Autodesk Inventor part; units mm, degrees
ref_plane "YZ Plane" through (0, 0, 0) normal (1, 0, 0) x (0, 1, 0)
ref_plane "XZ Plane" through (0, 0, 0) normal (0, 1, 0) x (-1, 0, 0)
ref_plane "XY Plane" through (0, 0, 0) normal (0, 0, 1) x (1, 0, 0)
sketch "Sketch1" plane through (0, 0, 0) normal (0, 0, 1) x (1, 0, 0)
  line L0 (-73.5219, 27.2789) -> (440.7773, 27.2789)
  line L1 (440.7773, 27.2789) -> (440.7773, -861.7211)
  line L2 (440.7773, -861.7211) -> (-73.5219, -861.7211)
  line L3 (-73.5219, -861.7211) -> (-73.5219, 27.2789)
  point P0 (0, 0)
  dimension "d0" = 514.2992
  dimension "d1" = 889
extrude "Extrusion1" add sketch "Sketch1" along normal blind 6.35
sketch "Sketch3" plane through (0, 0, 6.35) normal (0, 0, 1) x (1, 0, 0)
  line L0 (-73.5219, 27.2789) -> (104.2781, 27.2789)
  line L1 (104.2781, 27.2789) -> (104.2781, -433.4771)
  line L2 (104.2781, -433.4771) -> (-73.5219, -433.4771)
  line L3 (-73.5219, -433.4771) -> (-73.5219, 27.2789)
  line L4 (440.7773, 27.2789) -> (262.9773, 27.2789)
  line L5 (262.9773, 27.2789) -> (262.9773, -433.4771)
  line L6 (262.9773, -433.4771) -> (440.7773, -433.4771)
  line L7 (440.7773, -433.4771) -> (440.7773, 27.2789)
  point P0 (0, 0)
  dimension "d4" = 177.8
  dimension "d5" = 460.756
  dimension "d6" = 177.8
  dimension "d7" = 460.756
extrude "Extrusion2" cut sketch "Sketch3" against normal blind 25.4
sketch "Sketch4" plane through (104.2781, 27.2789, 0) normal (0, 1, 0) x (1, 0, 0)
  line L0 (0, 0) -> (0, -6.35)
  line L1 (0, -6.35) -> (158.6992, -6.35)
  line L2 (158.6992, -6.35) -> (158.6992, 0)
  line L3 (0, 0) -> (158.6992, 0)
  point P0 (-104.2781, 0)
extrude "Extrusion3" add sketch "Sketch4" along normal blind 6.35
sketch "Sketch5" plane through (104.2781, 33.6289, 0) normal (0, 1, 0) x (1, 0, 0)
  line L0 (0, 0) -> (158.6992, 0)
  line L1 (0, -6.35) -> (0, 0)
  line L2 (158.6992, -6.35) -> (0, -6.35)
  line L3 (158.6992, 0) -> (158.6992, -6.35)
  point P0 (-104.2781, 0)
extrude "Extrusion4" cut sketch "Sketch5" against normal blind 6.35
sketch "Sketch6" plane through (104.2781, 27.2789, 0) normal (0, 1, 0) x (1, 0, 0)
  line L0 (0, -6.35) -> (0, 0)
  line L1 (158.6992, -6.35) -> (0, -6.35)
  line L2 (158.6992, 0) -> (158.6992, -6.35)
  line L3 (0, 0) -> (158.6992, 0)
  point P0 (-104.2781, 0)
extrude "Extrusion5" add sketch "Sketch6" along normal blind 6.35
sketch "Sketch7" plane through (0, 0, 0) normal (0, 0, -1) x (-1, 0, 0)
  line L0 (-440.7773, -861.7211) -> (73.5219, -861.7211)
  line L1 (-104.2781, 33.6289) -> (-262.9773, 33.6289)
  line L2 (-183.6277, -861.7211) -> (-183.6277, -362.9159)
  circle A0 centre (-183.6277, -362.9159) radius 2.3495
  point P0 (0, 0)
  dimension "d16" = 498.8052
  dimension "d17" = 4.699
extrude "Extrusion6" cut sketch "Sketch7" against normal blind 25.4
sketch "Sketch8" plane through (0, 0, 0) normal (0, 0, -1) x (-1, 0, 0)
  circle A0 centre (-183.6277, -362.9159) radius 2.3495
  line L0 (-104.2781, 33.6289) -> (-262.9773, 33.6289)
  line L1 (-183.6277, -362.9159) -> (-183.6277, -593.4209)
  circle A1 centre (-183.6277, -593.4209) radius 2.3495
  point P0 (0, 0)
  dimension "d20" = 230.505
  dimension "d21" = 4.699
extrude "Extrusion7" cut sketch "Sketch8" against normal blind 25.4 contours A1
sketch "Sketch9" plane through (0, 0, 0) normal (0, 0, -1) x (-1, 0, 0)
  circle A0 centre (-183.6277, -593.4209) radius 2.3495
  circle A1 centre (-183.6277, -362.9159) radius 2.3495
  line L0 (-104.2781, 33.6289) -> (-262.9773, 33.6289)
  line L1 (-183.6277, 33.6289) -> (-183.6277, -347.3711)
  circle A2 centre (-183.6277, -347.3711) radius 2.3495
  line L2 (-183.6277, -347.3711) -> (-183.6277, -362.9159)
  line L3 (-183.6277, -593.4209) -> (-183.6277, -577.8761)
  circle A3 centre (-183.6277, -577.8761) radius 2.3495
  point P0 (0, 0)
  dimension "d24" = 381
  dimension "d25" = 15.5448
extrude "Extrusion8" cut sketch "Sketch9" against normal blind 25.4 contours A3 | A2 L1 L2 | L2 L1 A2
sketch "Sketch10" plane through (0, 0, 0) normal (0, 0, -1) x (-1, 0, 0)
  circle A0 centre (-183.6277, -593.4209) radius 2.3495
  circle A1 centre (-183.6277, -362.9159) radius 2.3495
  point P0 (0, 0)
extrude "Extrusion9" add sketch "Sketch10" against normal blind 6.35
sketch "Sketch11" plane through (0, 0, 6.35) normal (0, 0, 1) x (1, 0, 0)
  line L0 (104.2781, -433.4771) -> (-73.5219, -433.4771)
  line L1 (-73.5219, -861.7211) -> (-73.5219, -433.4771)
  line L2 (440.7773, -861.7211) -> (-73.5219, -861.7211)
  line L3 (440.7773, -433.4771) -> (440.7773, -861.7211)
  line L4 (262.9773, 33.6289) -> (104.2781, 33.6289)
  line L5 (49.7648, -433.4771) -> (49.7648, -750.9771)
  line L6 (49.7648, -750.9771) -> (49.7648, -757.3271)
  line L7 (49.7648, -757.3271) -> (-73.5219, -757.3271)
  line L8 (49.7648, -757.3271) -> (440.7773, -757.3271)
  point P0 (0, 0)
  dimension "d30" = 317.5
  dimension "d31" = 6.35
extrude "Extrusion10" cut sketch "Sketch11" against normal blind 6.35 contours L7 L8 L3 L2 L1
sketch "Sketch12" plane through (0, 0, 0) normal (0, 0, -1) x (-1, 0, 0)
  line L0 (-440.7773, -433.4771) -> (-440.7773, -757.3271)
  circle A0 centre (-183.6277, -577.8761) radius 2.3495
  circle A1 centre (-183.6277, -347.3711) radius 2.3495
  line L1 (-183.6277, -347.3711) -> (-183.6277, -249.3271)
  line L2 (-183.6277, -577.8761) -> (-183.6277, -479.8321)
  circle A2 centre (-183.6277, -479.8321) radius 2.3495
  circle A3 centre (-183.6277, -249.3271) radius 2.3495
  point P0 (0, 0)
  dimension "d34" = 98.044
  dimension "d35" = 98.044
extrude "Extrusion11" cut sketch "Sketch12" against normal blind 6.35 contours A2 | A3
sketch "Sketch13" plane through (0, 0, 0) normal (0, 0, -1) x (-1, 0, 0)
  circle A0 centre (-183.6277, -577.8761) radius 2.3495
  circle A1 centre (-183.6277, -347.3711) radius 2.3495
  point P0 (0, 0)
extrude "Extrusion12" add sketch "Sketch13" against normal blind 6.35
sketch "Sketch14" plane through (0, 0, 6.35) normal (0, 0, 1) x (1, 0, 0)
  line L0 (262.9773, -433.4771) -> (262.9773, 33.6289)
  line L1 (104.2781, 33.6289) -> (262.9773, 33.6289)
  line L2 (262.9773, 33.6289) -> (262.9773, 14.5789)
  line L3 (262.9773, 14.5789) -> (104.2781, 14.5789)
  line L4 (104.2781, 14.5789) -> (104.2781, 33.6289)
  point P0 (0, 0)
  dimension "d40" = 19.05
extrude "Extrusion13" cut sketch "Sketch14" against normal blind 25.4
properties part number "front"
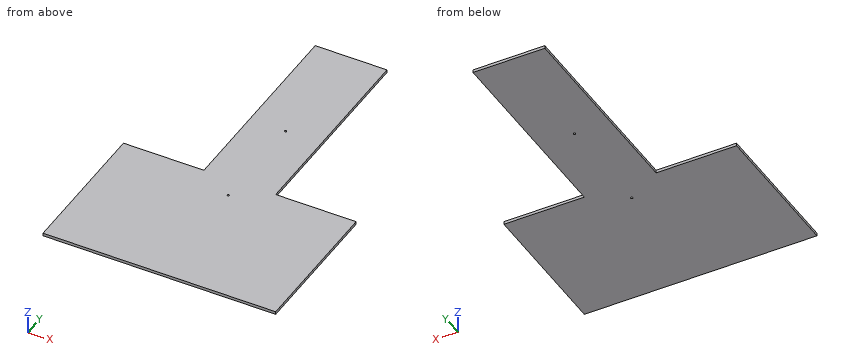
Part model, mm, in its own coordinate system. Round coordinates to 2 decimals unless told otherwise and drop trailing zeros. Order: outer loops, then holes, each group sorted by start corner. A loop starts at its lowest first (then second) coordinate and runs counter-clockwise, first axis right, second up. Notation, with made-up numbers: M -22,11.25 L 28,11.25 A28 ccw 28,29.25 Z; hole C 46,-4 d10. An arc over 180 degrees is marked long. Answer in a Markdown table with one row per item. Add a question column.
Q1. Wall check: L1, parallel to Y at x = 384.5, z = 4; L2, parallel to X at y = -336.5, z = 1. Give the ranges that are in metal, low to high. Write a range as from..to.
Q2. Cut at B-B on y = -175. Give the cut face in (x, z).
Q3. Pin check, flat tips, straight feed: pin 1 (6 mm diameter, centred on x = 183.63, y = -249.33, fed in from -Z); pin 2 (1.9 mm diameter, centred on y = -167.5, z = 3.5, fed in from +X); pin 3 (1.9 mm diameter, centred on x = 376.5, z = 2, fed in from +Y). Stop position of each tip, or through.
Q4. Cut at C-C on x = -39.5. Give the cut face in (y, z), and give its area (3 significant figures).
Q5. Cut at A-A on z = 1.75. Give the cut face in (x, y), and give its area (3 significant figures).
Established:
| question | item | result |
|---|---|---|
| 1 | L1 | y = -757.33..-433.48 |
| 1 | L2 | x = 104.28..262.98 |
| 2 | outline | M 104.28,0 L 262.98,0 L 262.98,6.35 L 104.28,6.35 Z |
| 3 | pin 1 | stops at z = 0 |
| 3 | pin 2 | stops at x = 262.98 |
| 3 | pin 3 | stops at y = -433.48 |
| 4 | outline | M -757.33,0 L -433.48,0 L -433.48,6.35 L -757.33,6.35 Z |
| 4 | area | 2,060 mm2 |
| 5 | outline | M -73.52,-757.33 L 440.78,-757.33 L 440.78,-433.48 L 262.98,-433.48 L 262.98,14.58 L 104.28,14.58 L 104.28,-433.48 L -73.52,-433.48 Z; hole C 183.63,-479.83 d4.7; hole C 183.63,-249.33 d4.7 |
| 5 | area | 238,000 mm2 |
